from build123d import *

# Parameters (mm, degrees)
F0_R     = 11.5
F0_R_2   = 10.5
F1_DEPTH = 203.2
F2_DEPTH = 25.4
F3_R     = 2.5019
F4_DEPTH = 12.7


with BuildPart() as f1:
    # F0 (on Front) → F1 (new body)
    with BuildSketch(Plane.XZ):
        Circle(F0_R)
        Circle(F0_R_2, mode=Mode.SUBTRACT)
        Circle(F0_R_2)
    extrude(amount=-F1_DEPTH)

    # F0 (on Front) → F2 (cut)
    with BuildSketch(Plane.XZ):
        Circle(F0_R_2)
    extrude(amount=-F2_DEPTH, mode=Mode.SUBTRACT)

    # F3 (on Right) → F4 (cut, symmetric)
    with BuildSketch(Plane.YZ):
        with Locations((12.7, 0)):
            Circle(F3_R)
    extrude(amount=F4_DEPTH, both=True, mode=Mode.SUBTRACT)


solid = f1.part
CAD build for the part. Positions are in the model's coordinates, mm. A direction names the side the tool comes from. Give positions to 0.01 mm unless a question says otherwise; leave off trailing zeros. Write each loop counter-clockwise with the first axis right and the second up, starting at its lowest first coordinate (ties: lowest second). Pieces come first, ordered by that corner, then holes. Notation, with made-up numbers: M 89.25,-4 L 147.25,-4 A10 ccw 147.25,6 Z; hole C 29.5,-0.5 d3. An arc over 180 degrees is marked long. Put each result on its own line as item: value. Start each with the question number.
(1) Band-saw the part on A-A, the plane z = 0. Write the cut outline in (x, y), and give its area (3 significant figures).
(2) Flat gauge pins, fed straight in: pin 1 Ø8 at (x, z) = (-3.5, -9) entering from -Y; pin 2 Ø5 at (y, z) = (162.5, -5) entering from +X (3 decimals); pin 3 Ø5 at (x, y) = (-8.5, 50) entering from +Z; pin 4 Ø6 at (x, y) = (7, 126) entering from -Z. Where does each tip first touch, or does it go through?
(3) Mould opens along Z. For faces 3 (the face through (-1.5, 100.2, 11.4)), 4 (the face through (0, 25.4, 0)), 5 (the face through (0, 203.2, 0)) say: +Z half, -Z half, draft (parallel to the pull), parting line (faces both ways), or undercut.
(4) Probe L1, parallel to Z at x = 0, y = 8.25; L2, parallel to X at y = 30, z = 0.75. List the from-to ranges inside material, lowest first.
(5) Band-saw the part on C-C, the plane y = 12.7. Write the cut outline in (x, z).
(6) Band-saw the part on B-B, the plane x = 0. Write the cut outline in (y, z), and give its area (3 significant figures).
(7) Which spindle directions (+Z, -Z, +X, -X, +Y, -Y) get a long thin tool onto all of the face, cutting with end or side? Do faces 1 (the face through (10.9, 10.2, 0.1)), 2 (the face through (10, 12.5, 3.2)). Say none if no direction does.
(8) Band-saw the part on D-D, the plane y = 179. Write the cut outline in (x, z).
Response values:
1. outline: M -11.5,0 L -10.5,0 L -10.5,10.2 L -11.5,10.2 Z; M -11.5,15.2 L -10.5,15.2 L -10.5,25.4 L 10.5,25.4 L 10.5,15.2 L 11.5,15.2 L 11.5,203.2 L -11.5,203.2 Z; M 10.5,0 L 11.5,0 L 11.5,10.2 L 10.5,10.2 Z
1. area: 4,130 mm2
2. pin 1: stops at y = 0
2. pin 2: stops at x = 11.225
2. pin 3: stops at z = 9.81
2. pin 4: stops at z = -10.78
3. face 3: parting line
3. face 4: undercut
3. face 5: draft
4. L1: z = -11.5 to -10.5, 10.5 to 11.5
4. L2: x = -11.48 to 11.48
5. outline: M -11.22,-2.5 A11.5 ccw 11.22,-2.5 L 10.2,-2.5 A10.5 cw -10.2,-2.5 Z; M -11.22,2.5 L -10.2,2.5 A10.5 cw 10.2,2.5 L 11.22,2.5 A11.5 ccw Z
6. outline: M 0,-11.5 L 203.2,-11.5 L 203.2,11.5 L 0,11.5 L 0,10.5 L 25.4,10.5 L 25.4,-10.5 L 0,-10.5 Z
6. area: 4,140 mm2
7. face 1: +X, -X
7. face 2: -Y
8. outline: C 0,0 d23
